Verification items for the finished model (mm, model axes). A direction names the side the tool comes from. Coordinates: 2 decimals unless noted, no trailing zeros. Loops run counter-clockwise (first coordinate to the right, second up) from the corner with the lowest first, then second, coordinate; pieces in that order, holes last.
Q1. Sectioned sample at C-C (y = 33.5). Enter the section's corners in (x, z), then the cut area to 3 significant figures.
Q2. Material ranges on probe 1 along Y at (x, z) = (0, 41); probe 2 along Z at (x, y) = (1, 21); probe 3 along Y at (x, z) = (-31, -37.5), recorded low to high.
Q3. Sectioned sample at B-B (x = 0). Count the separate pieces of the cut face and the enclosed holes in it, then the cut area to 3 significant figures.
Q4. Mould release check, pull along X, two halves, no side actions. Record for faces 1 (the face through (7.21, 61.21, 22.89)), 2 (the face through (7.21, 49.71, 22.89)), 3 (the face through (-32, 0, -17)), 4 (the face through (-44.835, 56.605, -45.671)): +X half, -X half, draft (parallel to the pull), parting line (faces both ways), or undercut.
Q5. Sectioned sample at D-D (y = 5.5). Enter the section's corners in (x, z), then the cut area to 3 significant figures.
Q6. Go/stop test with flat-tipped pins: P1, Ø12, axis at x = -0.5, y = 55, coming from the +Z side; P2, Ø5, axis at y = 32.5, z = -24, coming from the +X side; P3, Ø5, axis at x = 46, z = 33, coming from the -Y side; P4, Ø2.5, axis at x = 0, y = 18, coming from the +Z side. Record where each tip stops, or that it passes through.
Q7. Access from +Z, -Z, +X, -X, +Y, -Y to the whole of each face (thin tool, end or side, straight path). Record for faces 5 (the face through (59, 57, 8)), 6 (the face through (-8, 57, -59)), 7 (the face through (1.32, 55.73, -29.97)), 8 (the face through (10.81, 23.17, 34.34)).
```python
from build123d import *

# Parameters (mm, degrees)
SKETCH_1_W                = 64
SKETCH_1_H                = 15
CUT_EXTRUDE_1_DEPTH       = 92.744209627
CUT_EXTRUDE_2_DEPTH       = 92.744209627
CUT_EXTRUDE_3_DEPTH       = 92.744209627
CUT_EXTRUDE_4_DEPTH       = 92.394748208
HOLE_WIZARD_4_0_4_1_D     = 4
HOLE_WIZARD_4_0_4_1_DEPTH = 27.553629954
HOLE_WIZARD_4_0_4_2_D     = 4
HOLE_WIZARD_4_0_4_2_DEPTH = 108.498031466
CHAMFER_1_SIZE            = 2
CHAMFER_2_SIZE            = 1


with BuildPart() as part:
    # Эскиз1 → Повернуть1 (revolve)
    with BuildSketch(Plane(origin=(0, 0, 0), x_dir=(-1, 0, 0), z_dir=(0, 0, -1)), mode=Mode.PRIVATE) as revolve_1_sk:
        with Locations((-32, 56.5)):
            Rectangle(SKETCH_1_W, SKETCH_1_H)
    revolve(revolve_1_sk.sketch.rotate(Axis((0, 49, 0), (0, 1, 0)), 270), axis=Axis((0, 49, 0), (0, 1, 0)))

    # Эскиз2 → Вырез-Вытянуть1 (cut, through all)
    with BuildSketch(Plane(origin=(0, 64, 0), x_dir=(-1, 0, 0), z_dir=(0, 1, 0))):
        with BuildLine():
            Line((63.498031466, 8), (55, 8))
            Line((55, 8), (55, -8))
            Line((55, -8), (63.498031466, -8))
            ThreePointArc((63.498031466, -8), (64, 0), (63.498031466, 8))
        make_face()
    extrude(amount=-CUT_EXTRUDE_1_DEPTH, mode=Mode.SUBTRACT)

    # Эскиз3 → Вырез-Вытянуть2 (cut, through all)
    with BuildSketch(Plane(origin=(0, 64, 0), x_dir=(-1, 0, 0), z_dir=(0, 1, 0))):
        with BuildLine():
            Line((8, -63.498031466), (8, -55))
            Line((8, -55), (-8, -55))
            Line((-8, -55), (-8, -63.498031466))
            ThreePointArc((-8, -63.498031466), (0, -64), (8, -63.498031466))
        make_face()
    extrude(amount=-CUT_EXTRUDE_2_DEPTH, mode=Mode.SUBTRACT)

    # Эскиз4 → Вырез-Вытянуть3 (cut, through all)
    with BuildSketch(Plane(origin=(0, 64, 0), x_dir=(-1, 0, 0), z_dir=(0, 1, 0))):
        with BuildLine():
            Line((-63.498031466, -8), (-55, -8))
            Line((-55, -8), (-55, 8))
            Line((-55, 8), (-63.498031466, 8))
            ThreePointArc((-63.498031466, 8), (-64, 0), (-63.498031466, -8))
        make_face()
    extrude(amount=-CUT_EXTRUDE_3_DEPTH, mode=Mode.SUBTRACT)

    # Эскиз5 → Вырез-Вытянуть4 (cut, through all)
    with BuildSketch(Plane(origin=(0, 64, 0), x_dir=(-1, 0, 0), z_dir=(0, 1, 0))):
        with BuildLine():
            Line((-8, 63.498031466), (-8, 55))
            Line((-8, 55), (8, 55))
            Line((8, 55), (8, 63.498031466))
            ThreePointArc((8, 63.498031466), (0, 64), (-8, 63.498031466))
        make_face()
    extrude(amount=-CUT_EXTRUDE_4_DEPTH, mode=Mode.SUBTRACT)

    # Эскиз6 → Повернуть2 (revolve)
    with BuildSketch(Plane(origin=(0, 0, 0), x_dir=(-1, 0, 0), z_dir=(0, 0, -1)), mode=Mode.PRIVATE) as revolve_2_sk:
        Polygon((-45, 0), (0, 0), (0, 49), (-48, 49), (-48, 44), (-52, 44), (-52, 26), (-45, 26), align=None)
    revolve(revolve_2_sk.sketch.rotate(Axis((0, 0, 0), (0, 1, 0)), 270), axis=Axis((0, 0, 0), (0, 1, 0)))

    # Эскиз7 → Вырез-Повернуть1 (revolve, cut)
    with BuildSketch(Plane(origin=(0, 0, 0), x_dir=(-1, 0, 0), z_dir=(0, 0, -1)), mode=Mode.PRIVATE) as cut_revolve_1_sk:
        Polygon((-36, 0), (0, 0), (0, 64), (-24, 64), (-24, 58.5), (-30, 57.5), (-30, 54), (-24, 52.5), (-24, 47), (-36, 47), align=None)
    revolve(cut_revolve_1_sk.sketch.rotate(Axis((0, 0, 0), (0, 1, 0)), 270), axis=Axis((0, 0, 0), (0, 1, 0)), mode=Mode.SUBTRACT)

    # Диаметр отверстия Ø4.0 (4)1
    with Locations(Plane.XY.offset(-35.944401511)):
        with Locations((0, 18)):
            Hole(HOLE_WIZARD_4_0_4_1_D / 2, depth=HOLE_WIZARD_4_0_4_1_DEPTH)

    # Диаметр отверстия Ø4.0 (4)2
    with Locations(Plane(origin=(0, 18, 45), x_dir=(1, 0, 0), z_dir=(0, 0, 1))):
        with Locations((0, 0)):
            Hole(HOLE_WIZARD_4_0_4_2_D / 2, depth=HOLE_WIZARD_4_0_4_2_DEPTH)

    # Фаска1
    chamfer_1_edges = [part.edges().sort_by_distance(p)[0] for p in [
        (0, 26, -52),
    ]]
    chamfer(chamfer_1_edges, length=CHAMFER_1_SIZE)

    # Фаска2
    chamfer_2_edges = [part.edges().sort_by_distance(p)[0] for p in [
        (0, 0, -45),
    ]]
    chamfer(chamfer_2_edges, length=CHAMFER_2_SIZE)


solid = part.part
```
Geometry check:
1. outline: circle Ø104 at (0, 0); hole circle Ø72 at (0, 0)
1. area: 4,420 mm2
2. probe 1: y = 0 to 16, 20 to 64
2. probe 2: z = -44.99 to -35.99, 35.99 to 44.99
2. probe 3: y = 26 to 44, 49 to 64
3. separate pieces: 4
3. enclosed holes: 0
3. area: 2,010 mm2
4. face 1: undercut
4. face 2: undercut
4. face 3: draft
4. face 4: -X half
5. outline: circle Ø90 at (0, 0); hole circle Ø72 at (0, 0)
5. area: 2,290 mm2
6. P1: stops at z = 55
6. P2: stops at x = 47.35
6. P3: stops at y = 49
6. P4: passes through
7. face 5: +X, +Y, -Y
7. face 6: -Z, +Y, -Y
7. face 7: none
7. face 8: -Y
